Can you work these out from the drawing? Everything is in mm from the part's minimum corner. A direction names the side the tool comes from. Coordinates: 2 decimals unless noted, no trailing zeros. Order: outer loops, then holes, each group sorted by start corner. A loop starts at its lowest first (then second) coordinate and runs counter-clockwise, first axis right, second up. Notation, with made-up numbers: (-35, 51) -> (7, 51) arc R8 cw to (7, 56) -> close; hole circle Ø7 at (83, 43). An arc over 180 degrees is marked (long way). Put each result on its own line as item: value. Start each with the question number.
Q1. For the marked faces 1 and 2, which set-ups out of +Z, -Z, +X, -X, +Y, -Y let a thin tool reach every point of the face, with its end or its side?
Q2. We'd pull the mould along X, two halves only. Please class the marked faces 3, 4, 5 and 6: +X half, -X half, draft (parallel to the pull), parting line (faces both ways), or undercut.
Q3. If we section it at C-C (y = 2): Please give me the cut outline in (x, z), and give its area (3 significant figures).
Q4. If we section it at B-B (x = 8.5): Please give me the cut outline in (y, z).
Q5. If we section it at D-D (x = 6): Please give me the cut outline in (y, z).
Q6. Please list where these lines run through material, in increasing order: line 1 along Y through (x, z) = (3.5, 17); line 2 along X through (y, z) = (1.25, 32); line 3 along Y through (x, z) = (0.5, 27).
Q7. If we section it at A-A (z = 15): Please give me the cut outline in (x, y), and give its area (3 significant figures).
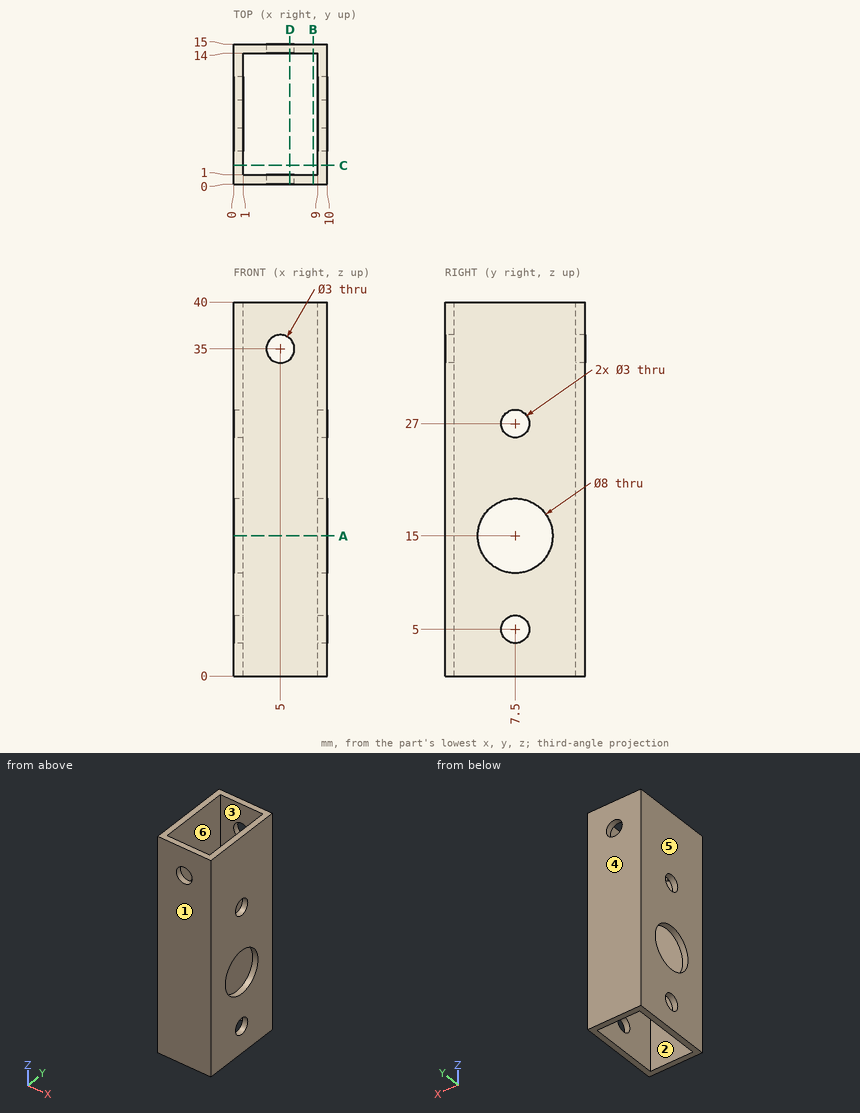
The answers:
1. face 1: +Z, -Z, +X, -X, -Y
1. face 2: +Z, -Z
2. face 3: undercut
2. face 4: draft
2. face 5: -X half
2. face 6: undercut
3. outline: (0, 0) -> (1, 0) -> (1, 40) -> (0, 40) -> close; (9, 0) -> (10, 0) -> (10, 40) -> (9, 40) -> close
3. area: 80.0 mm^2
4. outline: (0, 0) -> (1, 0) -> (1, 40) -> (0, 40) -> close; (14, 0) -> (15, 0) -> (15, 40) -> (14, 40) -> close
5. outline: (0, 0) -> (1, 0) -> (1, 33.88) -> (0, 33.88) -> close; (0, 36.12) -> (1, 36.12) -> (1, 40) -> (0, 40) -> close; (14, 0) -> (15, 0) -> (15, 33.88) -> (14, 33.88) -> close; (14, 36.12) -> (15, 36.12) -> (15, 40) -> (14, 40) -> close
6. line 1: 0 to 1, 14 to 15
6. line 2: 0 to 1, 9 to 10
6. line 3: 0 to 6, 9 to 15
7. outline: (0, 0) -> (10, 0) -> (10, 3.5) -> (9, 3.5) -> (9, 1) -> (1, 1) -> (1, 3.5) -> (0, 3.5) -> close; (0, 11.5) -> (1, 11.5) -> (1, 14) -> (9, 14) -> (9, 11.5) -> (10, 11.5) -> (10, 15) -> (0, 15) -> close
7. area: 30.0 mm^2
